from build123d import *

# Parameters (mm, degrees)
SKETCH1_W           = 141.104496432
SKETCH1_H           = 70.279121138
BOSS_EXTRUDE1_DEPTH = 50
SKETCH2_W           = 67.805568122
SKETCH2_H           = 49.81527963
SKETCH2_W_2         = 59.592894194
SKETCH2_H_2         = 42.894286786
BOSS_EXTRUDE2_DEPTH = 2
SKETCH3_R           = 7.50966637
SKETCH3_R_2         = 7.194748193
BOSS_EXTRUDE3_DEPTH = 4
SKETCH4_R           = 4.364569168
BOSS_EXTRUDE4_DEPTH = 10
SKETCH5_R           = 3.693674176
BOSS_EXTRUDE5_DEPTH = 15


with BuildPart() as part:
    # Sketch1 → Boss-Extrude1 (new body)
    with BuildSketch(Plane.XY):
        Rectangle(SKETCH1_W, SKETCH1_H)
    extrude(amount=BOSS_EXTRUDE1_DEPTH)

    # Sketch2 → Boss-Extrude2 (add)
    with BuildSketch(Plane.XY.offset(50)):
        with Locations((-27.427958915, 0)):
            Rectangle(SKETCH2_W, SKETCH2_H)
        with Locations((-27.077866503, 0)):
            Rectangle(SKETCH2_W_2, SKETCH2_H_2, mode=Mode.SUBTRACT)
    extrude(amount=BOSS_EXTRUDE2_DEPTH)

    # Sketch3 → Boss-Extrude3 (add)
    with BuildSketch(Plane.XY.offset(50)):
        with Locations((41.743235824, 16.179657371)):
            Circle(SKETCH3_R)
        with Locations((41.743235824, -13.592283792)):
            Circle(SKETCH3_R_2)
    extrude(amount=BOSS_EXTRUDE3_DEPTH)

    # Sketch4 → Boss-Extrude4 (add)
    with BuildSketch(Plane(origin=(70.552248216, 0, 0), x_dir=(0, 0, -1), z_dir=(1, 0, 0))):
        with Locations(Location((-13.969787954, 2.76951533, 0), (0, 0, 180))):
            Circle(SKETCH4_R)
    extrude(amount=BOSS_EXTRUDE4_DEPTH)

    # Sketch5 → Boss-Extrude5 (add)
    with BuildSketch(Plane(origin=(70.552248216, 0, 0), x_dir=(0, 0, -1), z_dir=(1, 0, 0))):
        with Locations(Location((-15.390317834, -20.981701915, 0), (0, 0, 180))):
            Circle(SKETCH5_R)
    extrude(amount=BOSS_EXTRUDE5_DEPTH)


solid = part.part
CAD build for the part. Positions are in the model's coordinates, mm. A direction names the side the tool comes from. Give positions to 0.01 mm unless a question says otherwise; leave off trailing zeros. Write each loop counter-clockwise with the first axis right and the second up, starting at its lowest first coordinate (ties: lowest second). Pieces come first, ordered by that corner, then holes. Notation, with made-up numbers: M -16,10 L 34,10 A16 cw 34,29 Z; hole C 46.5,84 d11. An arc over 180 degrees is marked long. Put each result on its own line as item: value. Start each with the question number.
(1) Mould opens along X. For faces 1 (the face through (-70.552, 0, 25)), 2 (the face through (80.552, 3, 14)), 3 (the face through (34.555, -13.276, 51.972)), 4 (the face through (-1, 35.14, 25)) say: +X half, -X half, draft (parallel to the pull), parting line (faces both ways), or undercut.
(2) Probe L1, parallel to Z at x = -3, y = -24; L2, parallel to X at y = -16, z = 48.5; L3, parallel to Z at x = 14.5, y = -24.5. List the from-to ranges inside material, lowest first.
(3) Band-saw the part on A-A, the plane x = -11.5. Write the cut outline in (y, z), and give its area (3 significant figures).
(4) Band-saw the part on D-D, the plane z = 38.5. Write the cut outline in (x, y), and give its area (3 significant figures).
(5) Band-saw the part on C-C, the plane x = 75. Write the cut outline in (y, z), and give its area (3 significant figures).
(6) Band-saw the part on B-B, the plane y = -3.5. Write the cut outline in (x, z), and give its area (3 significant figures).
(7) Flat gauge pins, fed straight in: pin 1 Ø0.6 at (x, z) = (-25.5, 51) entering from -Y; pin 2 Ø6 at (y, z) = (22, 20.5) entering from +X; pin 3 Ø1.6 at (x, z) = (-12.5, 51) entering from +Y. Where does each tip first touch, or does it go through?
(8) Which spindle directions (+Z, -Z, +X, -X, +Y, -Y) get a long thin tool onto all of the face, cutting with end or side? Do faces 5 (the face through (77.947, -22.091, 18.913)), 6 (the face through (-35, -22, 52)), 7 (the face through (45.8, 22.5, 52)), 8 (the face through (42, -13, 54)). Say none if no direction does.
Response values:
1. face 1: -X half
1. face 2: +X half
1. face 3: undercut
1. face 4: draft
2. L1: z = 0 to 52
2. L2: x = -70.55 to 70.55
2. L3: z = 0 to 50
3. outline: M -35.14,0 L 35.14,0 L 35.14,50 L 24.91,50 L 24.91,52 L 21.45,52 L 21.45,50 L -21.45,50 L -21.45,52 L -24.91,52 L -24.91,50 L -35.14,50 Z
3. area: 3,530 mm2
4. outline: M -70.55,-35.14 L 70.55,-35.14 L 70.55,35.14 L -70.55,35.14 Z
4. area: 9,920 mm2
5. outline: C -20.98,15.39 d7.39; C 2.77,13.97 d8.73
5. area: 103 mm2
6. outline: M -70.55,0 L 70.55,0 L 70.55,50 L 6.47,50 L 6.47,52 L 2.72,52 L 2.72,50 L -56.87,50 L -56.87,52 L -61.33,52 L -61.33,50 L -70.55,50 Z
6. area: 7,070 mm2
7. pin 1: stops at y = -24.91
7. pin 2: stops at x = 70.55
7. pin 3: stops at y = 24.91
8. face 5: +X
8. face 6: +Z, -X, +Y, -Y
8. face 7: +Z
8. face 8: +Z, +X, -X, +Y, -Y
